Part model, mm, in its own coordinate system. A direction names the side the tool comes from. Round coordinates to 2 decimals unless told otherwise and drop trailing zeros. Loops run counter-clockwise (first coordinate to the right, second up) from the corner with the lowest first, then second, coordinate; pieces in that order, holes last. Notation, with made-up numbers: M 47.25,8.25 L 104.25,8.25 A26 ccw 104.25,30.25 Z; hole C -32,-7.5 d2. An arc over 180 degrees is marked long. Write each question's results on one line, items separated by ' | '.
from build123d import *

# Parameters (mm, degrees)
DODANIE_WYCI_GNI_CIE2_DEPTH = 420
SZKIC4_R                    = 4.1
DODANIE_WYCI_GNI_CIE3_DEPTH = 6
SZKIC6_R                    = 8.6
WYTNIJ_WYCI_GNI_CIE1_DEPTH  = 430.73945595
DODANIE_WYCI_GNI_CIE5_REACH = 431.739
SZKIC6_3_R                  = 13.5
SZKIC6_3_R_2                = 8.6


with BuildPart() as part:
    # Szkic3 → Dodanie-wyci_gni_cie2 (new body)
    with BuildSketch(Plane(origin=(0, 0, 0), x_dir=(0, 0, -1), z_dir=(1, 0, 0))):
        with BuildLine():
            Line((-13.6, -20), (13.6, -20))
            ThreePointArc((13.6, -20), (18.1254834, -18.1254834), (20, -13.6))
            Line((20, -13.6), (20, 13.6))
            ThreePointArc((20, 13.6), (18.1254834, 18.1254834), (13.6, 20))
            Line((13.6, 20), (-13.6, 20))
            ThreePointArc((-13.6, 20), (-18.1254834, 18.1254834), (-20, 13.6))
            Line((-20, 13.6), (-20, -13.6))
            ThreePointArc((-20, -13.6), (-18.1254834, -18.1254834), (-13.6, -20))
        make_face()
        with BuildLine():
            Line((-9.6, 16), (9.6, 16))
            ThreePointArc((9.6, 16), (14.1254834, 14.1254834), (16, 9.6))
            Line((16, 9.6), (16, -9.6))
            ThreePointArc((16, -9.6), (14.1254834, -14.1254834), (9.6, -16))
            Line((9.6, -16), (-9.6, -16))
            ThreePointArc((-9.6, -16), (-14.1254834, -14.1254834), (-16, -9.6))
            Line((-16, -9.6), (-16, 9.6))
            ThreePointArc((-16, 9.6), (-14.1254834, 14.1254834), (-9.6, 16))
        make_face(mode=Mode.SUBTRACT)
    extrude(amount=DODANIE_WYCI_GNI_CIE2_DEPTH)

    # Szkic4 → Dodanie-wyci_gni_cie3 (add)
    with BuildSketch(Plane(origin=(420, 0, 0), x_dir=(0, 0, -1), z_dir=(1, 0, 0))):
        with BuildLine():
            Line((-13.6, -40), (13.6, -40))
            ThreePointArc((13.6, -40), (18.1254834, -38.1254834), (20, -33.6))
            Line((20, -33.6), (20, 33.6))
            ThreePointArc((20, 33.6), (18.1254834, 38.1254834), (13.6, 40))
            Line((13.6, 40), (-13.6, 40))
            ThreePointArc((-13.6, 40), (-18.1254834, 38.1254834), (-20, 33.6))
            Line((-20, 33.6), (-20, -33.6))
            ThreePointArc((-20, -33.6), (-18.1254834, -38.1254834), (-13.6, -40))
        make_face()
        with Locations((0, 30)):
            Circle(SZKIC4_R, mode=Mode.SUBTRACT)
        with Locations(Location((0, -30, 0), (0, 0, 180))):
            Circle(SZKIC4_R, mode=Mode.SUBTRACT)
    dodanie_wyci_gni_cie3 = extrude(amount=DODANIE_WYCI_GNI_CIE3_DEPTH)

    # Lustro4: Dodanie-wyci_gni_cie3 across plane
    add(dodanie_wyci_gni_cie3.mirror(Plane(origin=(210, 0, 0), x_dir=(0, 0, 1), z_dir=(1, 0, 0))))

    # Szkic6 → Wytnij-wyci_gni_cie1 (cut, through all)
    with BuildSketch(Plane(origin=(0, 0, -20), x_dir=(-1, 0, 0), z_dir=(0, 0, -1))):
        with Locations((-40, 0)):
            Circle(SZKIC6_R)
    wytnij_wyci_gni_cie1 = extrude(amount=-WYTNIJ_WYCI_GNI_CIE1_DEPTH, mode=Mode.SUBTRACT)

    # Szkic6_3 → Dodanie-wyci_gni_cie5 (add, up to next)
    with BuildSketch(Plane(origin=(0, 0, -20), x_dir=(-1, 0, 0), z_dir=(0, 0, -1)), mode=Mode.PRIVATE) as dodanie_wyci_gni_cie5_sk1:
        with Locations(Location((-40, 0, 0), (0, 0, 314.674609564))):
            Circle(SZKIC6_3_R)
        with Locations((-40, 0)):
            Circle(SZKIC6_3_R_2, mode=Mode.SUBTRACT)
    dodanie_wyci_gni_cie5_tool1 = extrude(dodanie_wyci_gni_cie5_sk1.sketch, amount=-DODANIE_WYCI_GNI_CIE5_REACH, mode=Mode.PRIVATE) - part.part
    dodanie_wyci_gni_cie5 = dodanie_wyci_gni_cie5_tool1.solids().sort_by_distance((49.223113, 9.328471, -20))[0]
    add(dodanie_wyci_gni_cie5)

    # Lustro6: Wytnij-wyci_gni_cie1, Dodanie-wyci_gni_cie5 across plane
    add(wytnij_wyci_gni_cie1.mirror(Plane(origin=(210, 0, 0), x_dir=(0, 0, 1), z_dir=(1, 0, 0))), mode=Mode.SUBTRACT)
    add(dodanie_wyci_gni_cie5.mirror(Plane(origin=(210, 0, 0), x_dir=(0, 0, 1), z_dir=(1, 0, 0))))


solid = part.part
Item 1: Which spindle directions (+Z, -Z, +X, -X, +Y, -Y) get a long thin tool onto all of the face, cutting with end or side? Do faces 1 (the cylindrical face through (28.063, -6.306, -0.224)), 2 (the cylindrical face through (423, 26, 0.9)), 3 (the flat face through (207, -20, 0)). Say none if no direction does.
Filled sheet:
face 1: none | face 2: +X, -X | face 3: +Z, -Z, -Y
Item 2: Band-saw the part on B-B on x = 166.5. Give the cut face in (y, z), and give its area (3 significant figures).
Filled sheet:
outline: M -20,-13.6 A6.4 ccw -13.6,-20 L 13.6,-20 A6.4 ccw 20,-13.6 L 20,13.6 A6.4 ccw 13.6,20 L -13.6,20 A6.4 ccw -20,13.6 Z; hole M -16,-9.6 A6.4 ccw -9.6,-16 L 9.6,-16 A6.4 ccw 16,-9.6 L 16,9.6 A6.4 ccw 9.6,16 L -9.6,16 A6.4 ccw -16,9.6 Z | area: 576 mm^2
Item 3: Band-saw the part on C-C on z = 0. Count the separate pieces of the cut face and the enclosed holes in it, and give its area (3 significant figures).
Filled sheet:
separate pieces: 7 | enclosed holes: 3 | area: 4,800 mm^2
Item 4: Band-saw the part on D-D on y = 30. Give the cut face in (x, z).
Filled sheet:
outline: M -6,-20 L 0,-20 L 0,-4.1 L -6,-4.1 Z; M -6,4.1 L 0,4.1 L 0,20 L -6,20 Z; M 420,-20 L 426,-20 L 426,-4.1 L 420,-4.1 Z; M 420,4.1 L 426,4.1 L 426,20 L 420,20 Z
Item 5: Wall check: L1, parallel to Y at x = 40, z = 6; L2, parallel to Y at x = -3.9, z = 0; L3, parallel to Z at x = 404, y = 9. Give the ranges that are in metal, low to high.
Filled sheet:
L1: -20 to -16, -13.5 to -8.6, 8.6 to 13.5, 16 to 20 | L2: -40 to -34.1, -25.9 to 25.9, 34.1 to 40 | L3: -20 to -16, 16 to 20
Item 6: Drop flat-ended pins along their axis: P1, Ø15.5, axis at x = 380, y = 0, coming from the -Z side; P2, Ø10, axis at x = 361.5, z = -5, coming from the -Y side; P3, Ø12, axis at x = 282, y = 17.5, coming from the -Z side; P4, Ø6, axis at x = 214, z = 0.5, coming from the +Y side. Give the stop position or say it passes through.
Filled sheet:
P1: through | P2: y = -20 | P3: z = -20 | P4: y = 20
Item 7: Two-plate mould, pull along X, no slides. Class faces 4 (the flat face through (207, 20, 0)), 5 (the flat face through (211, 3, 20)), 6 (the flat face through (426, 1, 0)): +X half, -X half, draft (parallel to the pull), parting line (faces both ways), or undercut.
Filled sheet:
face 4: undercut | face 5: draft | face 6: +X half
Item 8: Band-saw the part on A-A on y = 0. Give the cut face in (x, z).
Filled sheet:
outline: M -6,-20 L 31.4,-20 L 31.4,20 L -6,20 Z; M 48.6,-20 L 371.4,-20 L 371.4,20 L 48.6,20 Z; M 388.6,-20 L 426,-20 L 426,20 L 388.6,20 Z; hole M 0,-16 L 26.5,-16 L 26.5,16 L 0,16 Z; hole M 53.5,-16 L 366.5,-16 L 366.5,16 L 53.5,16 Z; hole M 393.5,-16 L 420,-16 L 420,16 L 393.5,16 Z
